Input: part model. Units: mm. Frame: model coordinates. Give positions to 0.01 mm unless a question says otherwise; leave off trailing zeros. Loops run counter-clockwise (first coordinate to the right, second up) from the corner with the lowest first, then second, coordinate; pieces in that order, holes last. Notation, with made-up numbers: M -22.75,-2.5 L 33.25,-2.5 A24 cw 33.25,19.5 Z; hole C -3.5,20 d4. An arc over 180 degrees is marked long. Use a Markdown table: item, result. Add a question column.
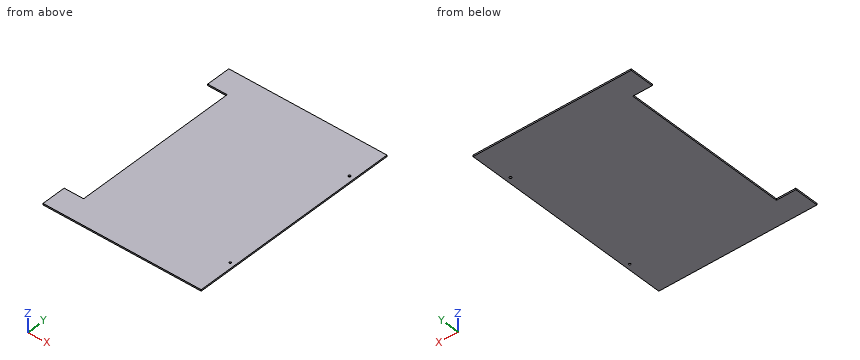
from build123d import *

# Parameters (mm, degrees)
SKETCH1_W           = 325
SKETCH1_H           = 70
SKETCH1_H_2         = 300
BOSS_EXTRUDE1_DEPTH = 3
SKETCH2_W           = 40
SKETCH2_H           = 340
CUT_EXTRUDE1_DEPTH  = 3
SKETCH3_R           = 2
SKETCH3_R_2         = 2.415919743
CUT_EXTRUDE2_DEPTH  = 3


with BuildPart() as part:
    # Sketch1 → Boss-Extrude1 (new body)
    with BuildSketch(Plane.XY):
        with Locations((16, 188.326300096)):
            Rectangle(SKETCH1_W, SKETCH1_H)
        with Locations((16, 3.326300096)):
            Rectangle(SKETCH1_W, SKETCH1_H_2)
        with Locations((16, -181.673699904)):
            Rectangle(SKETCH1_W, SKETCH1_H)
    extrude(amount=BOSS_EXTRUDE1_DEPTH)

    # Sketch2 → Cut-Extrude1 (cut)
    with BuildSketch(Plane.XY.offset(3)):
        with Locations((-126.5, 3.326300096)):
            Rectangle(SKETCH2_W, SKETCH2_H)
    extrude(amount=-CUT_EXTRUDE1_DEPTH, mode=Mode.SUBTRACT)

    # Sketch3 → Cut-Extrude2 (cut)
    with BuildSketch(Plane(origin=(0, 0, 0), x_dir=(-1, 0, 0), z_dir=(0, 0, -1))):
        with Locations((-168.5, -136.673699904)):
            Circle(SKETCH3_R)
        with Locations((-168.5, 146.326300096)):
            Circle(SKETCH3_R_2)
    extrude(amount=-CUT_EXTRUDE2_DEPTH, mode=Mode.SUBTRACT)


solid = part.part
1) Ray query, line 1 (Y direction, x = 168.5, z = 1.7); line 2 (X direction, y = 118, z = 1.55). Return the intervals inside material, ascending. Write a range as [from, to].
2) Section query B-B, the plane y = -117. Return the cut outline in (x, z), and give its area (3 significant figures).
3) Section query A-A, the plane z = 1.8. Return the cut outline in (x, y), and give its area (3 significant figures).
Entries:
| question | item | result |
|---|---|---|
| 1 | line 1 | y = [-216.67, -138.67], [-134.67, 143.91], [148.74, 223.33] |
| 1 | line 2 | x = [-106.5, 178.5] |
| 2 | outline | M -106.5,0 L 178.5,0 L 178.5,3 L -106.5,3 Z |
| 2 | area | 855 mm² |
| 3 | outline | M -146.5,-216.67 L 178.5,-216.67 L 178.5,223.33 L -146.5,223.33 L -146.5,173.33 L -106.5,173.33 L -106.5,-166.67 L -146.5,-166.67 Z; hole C 168.5,146.33 d4.83; hole C 168.5,-136.67 d4 |
| 3 | area | 129,000 mm² |
